Build history of the part. All positions in model axes, mm. Face numbers are marked on the shaded views. Give positions to 0.01 mm unless a question says otherwise; leave off trailing zeros. Loops run counter-clockwise (first coordinate to the right, second up) from the corner with the lowest first, then second, coordinate; pieces in that order, holes last.
1) Wall check: line 1 (X direction, y = -14.5, z = 18.5) (3 decimals); line 2 (X direction, y = -5.5, z = -73.5); line 3 (X direction, y = -2.5, z = -35.5). Give the ranges that are in metal, low to high.
2) Two-plate mould, pull along X, no slides. Class the marked faces 1, 2 and 3: +X half, -X half, draft (parallel to the pull), parting line (faces both ways), or undercut.
3) Band-saw the part on C-C on x = -77.5. List the corners of the cut face in (y, z), then the cut area to 3 significant figures.
4) Flat gauge pins, fed straight in: P1, Ø3, axis at y = -20.5, z = 28, coming from the +X side; P2, Ø2, axis at x = -21, y = -6, coming from the -Z side; P3, Ø5, axis at x = -15, y = -7, coming from the -Z side. Where does each tip first touch, or does it go through?
5) Band-saw the part on A-A on y = -8.75. State how many separate pieces and enclosed holes the cut face has, then the cut area to 3 significant figures.
6) Band-saw the part on D-D on x = -28. List the corners of the cut face in (y, z).
7) Band-saw the part on B-B on z = -82. List the corners of the cut face in (x, y), then the cut area to 3 significant figures.
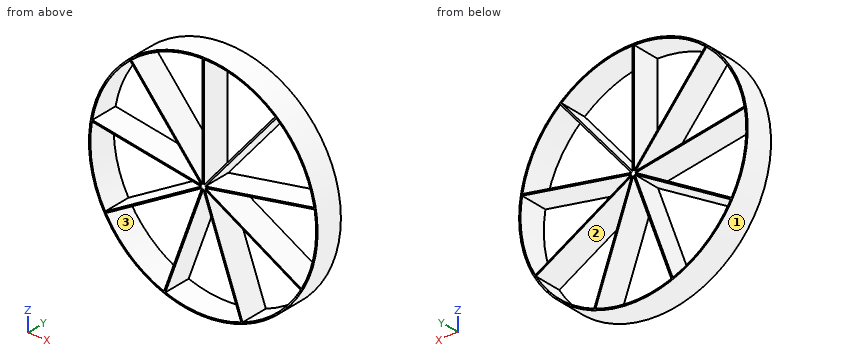
```python
from build123d import *

# Parameters (mm, degrees)
F0_R     = 102.235
F0_R_2   = 100.965
F1_DEPTH = 25.4
F2_W     = 1.27
F2_H     = 101.0406836867
F3_DEPTH = 25.4
F5_COUNT = 9


with BuildPart() as f1:
    # F0 (on Front) → F1 (new body)
    with BuildSketch(Plane.XZ):
        Circle(F0_R)
        Circle(F0_R_2, mode=Mode.SUBTRACT)
    extrude(amount=F1_DEPTH)



with BuildPart() as f3:
    # F2 (on Front) → F3 (new body)
    with BuildSketch(Plane.XZ):
        with Locations((0, 50.5203418434)):
            Rectangle(F2_W, F2_H)
    extrude(amount=F3_DEPTH)


with BuildPart() as f1_1:
    add(f1.part)

    add(f3.part)  # F5 merges F3
    # F5: F3 ×9 about axis
    f5_axis = Axis((0, 4.7910101712, 0), (0, 1, 0))
    for i in range(1, F5_COUNT):
        add(f3.part.rotate(f5_axis, i * 360 / F5_COUNT))


solid = f1_1.part
```
Findings below:
1. line 1: x = -100.547 to -99.256, -16.352 to -14.694, -0.635 to 0.635, 14.694 to 16.352, 99.256 to 100.547
1. line 2: x = -71.06 to -69.22, -27.43 to -26.08, 26.08 to 27.43, 69.22 to 71.06
1. line 3: x = -95.87 to -94.52, -62.76 to -60.22, -13.6 to -12.25, 12.25 to 13.6, 60.22 to 62.76, 94.52 to 95.87
2. face 1: parting line
2. face 2: undercut
2. face 3: undercut
3. outline: (-25.4, -66.68) - (0, -66.68) - (0, -64.71) - (-25.4, -64.71) - close; (-25.4, -45.48) - (0, -45.48) - (0, -44.01) - (-25.4, -44.01) - close; (-25.4, 13.02) - (0, 13.02) - (0, 14.31) - (-25.4, 14.31) - close; (-25.4, 64.71) - (0, 64.71) - (0, 66.68) - (-25.4, 66.68) - close
3. area: 170 mm2
4. P1: stops at x = 98.74
4. P2: stops at z = -100.26
4. P3: stops at z = -101.47
5. separate pieces: 1
5. enclosed holes: 9
5. area: 1,950 mm2
6. outline: (-25.4, -98.33) - (0, -98.33) - (0, -97) - (-25.4, -97) - close; (-25.4, -78.79) - (0, -78.79) - (0, -75.07) - (-25.4, -75.07) - close; (-25.4, -16.9) - (0, -16.9) - (0, -15.43) - (-25.4, -15.43) - close; (-25.4, 4.29) - (0, 4.29) - (0, 5.58) - (-25.4, 5.58) - close; (-25.4, 32.38) - (0, 32.38) - (0, 34.36) - (-25.4, 34.36) - close; (-25.4, 97) - (0, 97) - (0, 98.33) - (-25.4, 98.33) - close
7. outline: (-61.06, -25.4) - (-58.91, -25.4) - (-58.91, 0) - (-61.06, 0) - close; (-30.52, -25.4) - (-29.17, -25.4) - (-29.17, 0) - (-30.52, 0) - close; (29.17, -25.4) - (30.52, -25.4) - (30.52, 0) - (29.17, 0) - close; (58.91, -25.4) - (61.06, -25.4) - (61.06, 0) - (58.91, 0) - close
7. area: 178 mm2
